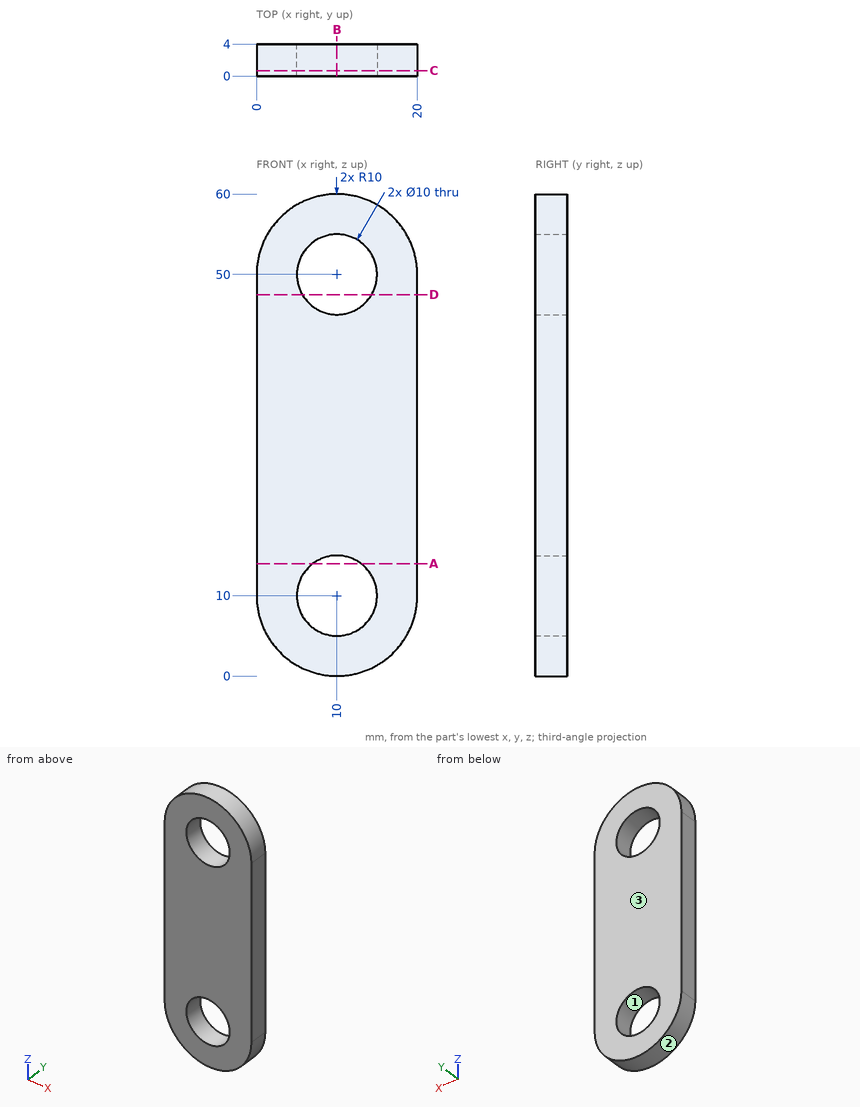
Input: dimensioned drawing with shaded views. Units: mm. Origin: part minimum x, y, z. Coordinates: 2 decimals unless noted, no trailing zeros. Write each loop counter-clockwise with the first axis right and the second up, starting at its lowest first coordinate (ties: lowest second). Pieces come first, ordered by that corner, then holes. Notation, with made-up numbers: M -9.5,-16 L -5.5,-16 A25 cw -5.5,4 Z; hole C 81.25,36.5 d2. An arc over 180 degrees is marked long. Answer as CSV lines item,"result". Start each with the question number.
Q1. Cut plane B-B on x = 10. Return the cut outline in (y, z).
Q2. Cut plane A-A on z = 14. Return the cut outline in (x, y), then the cut area to 3 significant figures.
Q3. Cut plane C-C on y = 0.7. Return the cut outline in (x, z).
Q4. Mould query, pull axis Z, two halves, no side actions, for the marked faces 1, 2 and 3. Classes: released by +Z, released by -Z, zero draft, split by the parting line, or undercut.
Q5. Cut plane D-D on z = 47.5. Return the cut outline in (x, y), then the cut area to 3 significant figures.
Q6. Line query: line 1 (Z direction, x = 10, y = 1.25); line 2 (Z direction, x = 14.5, y = 0.6); line 3 (X direction, y = 0.55, z = 6.5). Output: solid intervals per line, ascending. Write a range as from..to.
Findings below:
1,outline,"M 0,0 L 4,0 L 4,5 L 0,5 Z; M 0,15 L 4,15 L 4,45 L 0,45 Z; M 0,55 L 4,55 L 4,60 L 0,60 Z"
2,outline,"M 0,0 L 7,0 L 7,4 L 0,4 Z; M 13,0 L 20,0 L 20,4 L 13,4 Z"
2,area,"56.0 mm2"
3,outline,"M 0,10 A10 ccw 20,10 L 20,50 A10 ccw 0,50 Z; hole C 10,10 d10; hole C 10,50 d10"
4,face 1,"undercut"
4,face 2,"released by -Z"
4,face 3,"zero draft"
5,outline,"M 0,0 L 5.67,0 L 5.67,4 L 0,4 Z; M 14.33,0 L 20,0 L 20,4 L 14.33,4 Z"
5,area,"45.4 mm2"
6,line 1,"z = 0..5, 15..45, 55..60"
6,line 2,"z = 1.07..7.82, 12.18..47.82, 52.18..58.93"
6,line 3,"x = 0.63..6.43, 13.57..19.37"
